The figure shows three views and two pictorial views of one solid part (mm, origin at its lowest corner). Answer the questions. A direction names the side the tool comes from. Give positions to 0.01 mm unless a question says otherwise; leave off trailing zeros. Loops run counter-clockwise (first coordinate to the right, second up) from the corner with the lowest first, then second, coordinate; pieces in that order, holes last.
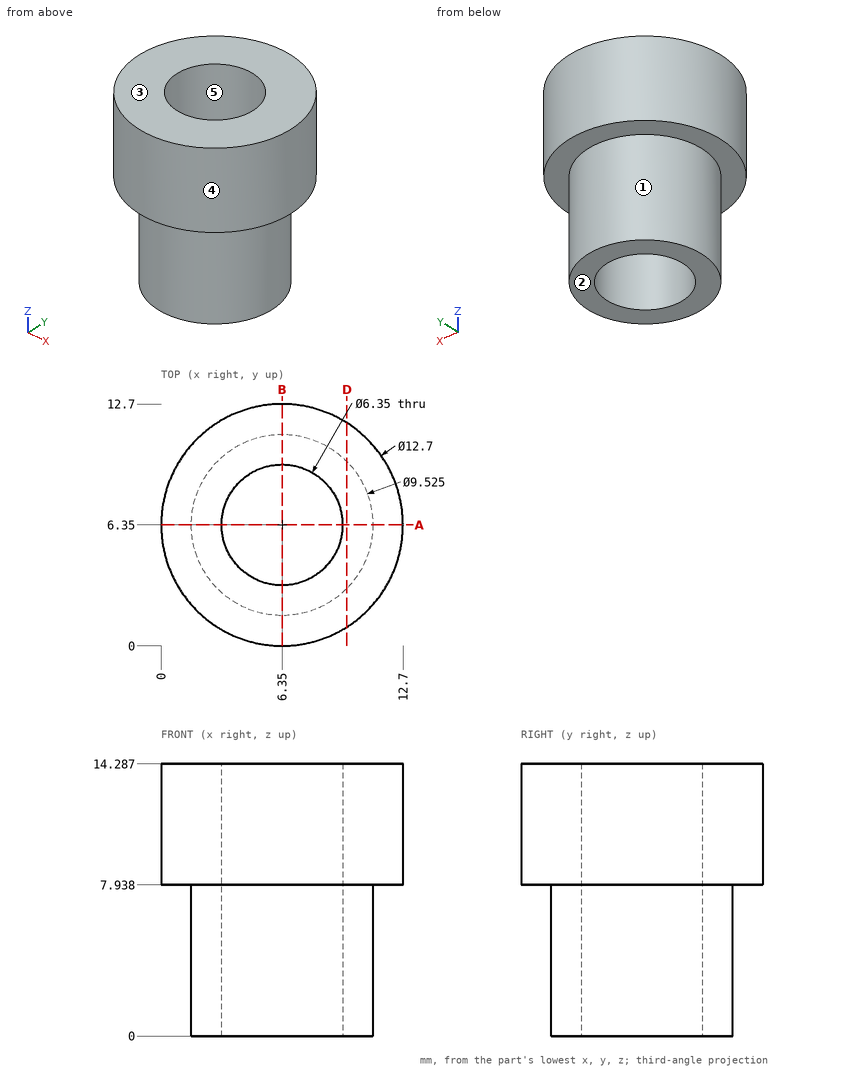
Q1. Consider line 1 along X through (y, z) = (6.5, 8.5); line 2 along Y through (x, z) = (6.35, 6.5) (1 decimal); line 3 along Z through (x, y) = (3.75, 11). Determine where each line is inside the solid, lowest interval first.
Q2. Section A-A on y = 6.35 is taken. Give the vertices of the cut face in (x, z) (1 decimal).
Q3. Which of the six approach directions +Z, -Z, +X, -X, +Y, -Y give full straight-line access (tool end or side, diameter ignored) to the marked faces 1 and 2?
Q4. Given pin 1 (1 mm diameter, centred on x = 1.5, z = 5.5, fed in from +Y) (1 decimal); pin 2 (1.5 mm diameter, centred on y = 9.5, z = 7.5, fed in from +X); pin 3 (2 mm diameter, centred on x = 8, z = 9, fed in from +Y), each flat-ended and moving along its own axis, determine where each tip first touches the part or whether it passes through.
Q5. Determine the mould class of the marked faces 3, 4 and 5 for opening direction X: +X half, -X half, draft (parallel to the pull), parting line (faces both ways), or undercut.
Q6. Section D-D on x = 9.75 is taken. Give the vertices of the cut face in (y, z) (1 decimal).
Check result:
1. line 1: x = 0 to 3.18, 9.52 to 12.7
1. line 2: y = 1.6 to 3.2, 9.5 to 11.1
1. line 3: z = 7.94 to 14.29
2. outline: (0, 7.9) - (1.6, 7.9) - (1.6, 0) - (3.2, 0) - (3.2, 14.3) - (0, 14.3) - close; (9.5, 0) - (11.1, 0) - (11.1, 7.9) - (12.7, 7.9) - (12.7, 14.3) - (9.5, 14.3) - close
3. face 1: -Z
3. face 2: -Z, +X, -X, +Y, -Y
4. pin 1: stops at y = 8.3
4. pin 2: stops at x = 12.17
4. pin 3: stops at y = 12.67
5. face 3: draft
5. face 4: parting line
5. face 5: undercut
6. outline: (1, 7.9) - (3, 7.9) - (3, 0) - (9.7, 0) - (9.7, 7.9) - (11.7, 7.9) - (11.7, 14.3) - (1, 14.3) - close
